Check sheet for the drawn part. Datum: minimum x, y, z corner. Units: mm. A direction names the side the tool comes from. Coordinates: 2 decimals unless noted, no trailing zeros. Order: outer loops, then holes, each group sorted by start corner. A loop starts at its lowest first (then second) coordinate and runs counter-clockwise, first axis right, second up. Notation, with made-up numbers: (74.5, 51) - (114.5, 51) arc R26 ccw to (114.5, 74) - close; hole circle Ø9 at (-5, -25). An arc over 180 degrees is marked (long way). One line per item, written item: value. Start each with the question number.
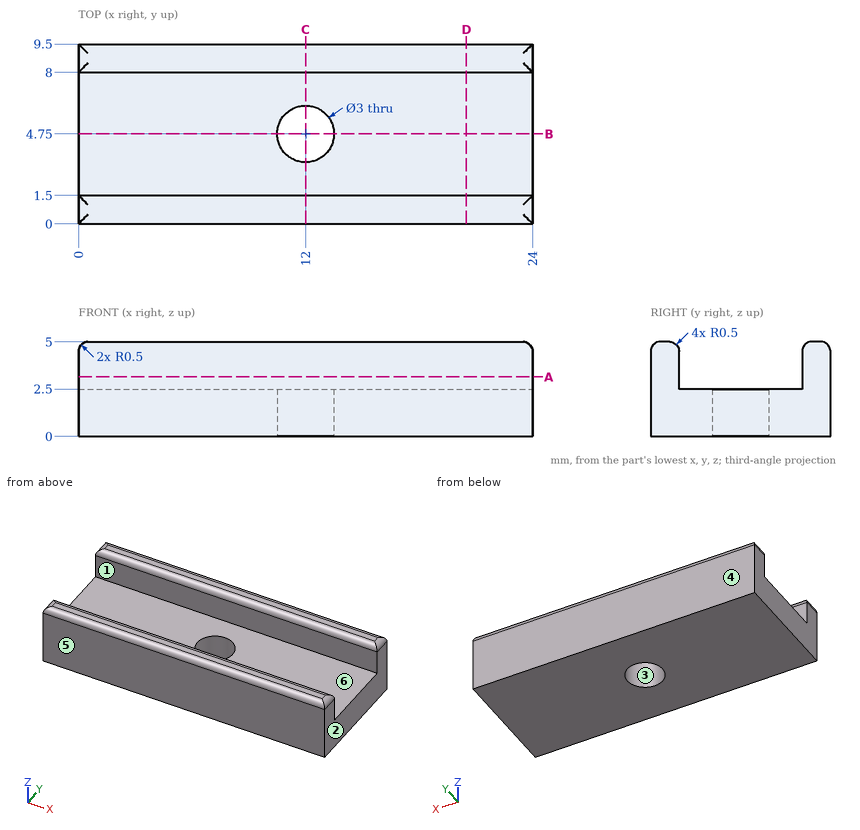
Q1. Cross-section at A-A, the plane z = 3.15. Enter the section's corners in (x, y).
Q2. Cross-section at D-D, the plane x = 20.5. Enter the section's corners in (y, z), and give its area (3 significant figures).
Q3. Release check for a two-part mould opening along Y. For the marked faces 1, 2, 3 and 4 record: released by +Y, released by -Y, zero draft, split by the parting line, or undercut.
Q4. Gauge pin test, flat ends, axial feed: P1, Ø3, axis at x = 7.5, y = 3.5, coming from the +Z side; P2, Ø1, axis at y = 4, z = 3.5, coming from the +X side. Record the tip position at first contact, or that the pin passes through.
Q5. Cross-section at C-C, the plane x = 12. Enter the section's corners in (y, z), and give its area (3 significant figures).
Q6. Material ranges on probe 1 along Y at (x, z) = (12, 1.15); probe 2 along Y at (x, z) = (1.75, 4.4); probe 3 along Z at (x, y) = (19, 5.5), recorded low to high.
Q7. Set-up check for the marked faces 5 and 6: record each of +Z, -Z, +X, -X, +Y, -Y from which the full face is reachable in a straight line by a thin tool's end or side.
Q8. Cross-section at B-B, the plane y = 4.75. Enter the section's corners in (x, z).
Check result:
1. outline: (0, 0) - (24, 0) - (24, 1.5) - (0, 1.5) - close; (0, 8) - (24, 8) - (24, 9.5) - (0, 9.5) - close
2. outline: (0, 0) - (9.5, 0) - (9.5, 4.5) arc R0.5 ccw to (9, 5) - (8.5, 5) arc R0.5 ccw to (8, 4.5) - (8, 2.5) - (1.5, 2.5) - (1.5, 4.5) arc R0.5 ccw to (1, 5) - (0.5, 5) arc R0.5 ccw to (0, 4.5) - close
2. area: 31.0 mm2
3. face 1: undercut
3. face 2: zero draft
3. face 3: undercut
3. face 4: released by +Y
4. P1: stops at z = 2.5
4. P2: passes through
5. outline: (0, 0) - (3.25, 0) - (3.25, 2.5) - (1.5, 2.5) - (1.5, 4.5) arc R0.5 ccw to (1, 5) - (0.5, 5) arc R0.5 ccw to (0, 4.5) - close; (6.25, 0) - (9.5, 0) - (9.5, 4.5) arc R0.5 ccw to (9, 5) - (8.5, 5) arc R0.5 ccw to (8, 4.5) - (8, 2.5) - (6.25, 2.5) - close
5. area: 23.5 mm2
6. probe 1: y = 0 to 3.25, 6.25 to 9.5
6. probe 2: y = 0 to 1.5, 8 to 9.5
6. probe 3: z = 0 to 2.5
7. face 5: +Z, -Z, +X, -X, -Y
7. face 6: +Z, +X, -X
8. outline: (0, 0) - (10.5, 0) - (10.5, 2.5) - (0, 2.5) - close; (13.5, 0) - (24, 0) - (24, 2.5) - (13.5, 2.5) - close
